Work out the finished part from the listing and answer in its coordinate system (mm). A direction names the side the tool comes from. Give positions to 0.01 mm unless a question says otherwise; leave off trailing zeros.
1) Straight lines are drawn through the part: probe 1 along Y at (x, z) = (0, 6.25) (3 decimals); probe 2 along X at (y, z) = (-9, 5.25); probe 3 along X at (y, z) = (8, 13). For each, find the intervals that lie inside material, in ascending order.
2) Determine the mould class of faces 1 (the face through (-12, 0, 14.1)), 2 (the face through (-19, 3, 12.6)), 3 (the face through (25.865, -10.724, 5.965)) for opening direction X: pulls with the +X half, pulls with the -X half, needs draft (parallel to the pull), parting line crosses it, or undercut.
3) Given pin 1 Ø1 at (y, z) = (-14.5, 11) entering from -X; pin 2 Ø2.5 at (x, y) = (6.5, -18) entering from +Z; pin 3 Ø5 at (y, z) = (-11.5, 11.5) entering from -X, each flat-ended and moving along its own axis, determine where each tip first touches the part or whether it passes through.
4) A tool of negligible diameter and unlimited length cuts with its end or side. For faces 4 (the face through (0, 20, 12.6)), 5 (the face through (-8.2, 7.52, 6.95)), from which of +Z, -Z, +X, -X, +Y, -Y can it reach the whole face along a straight path? Write none if from no direction.
```python
from build123d import *

# Parameters (mm, degrees)
F0_R     = 28
F0_R_2   = 11.125
F1_DEPTH = 14.1
F2_R     = 2
F3_R     = 5
F4_DEPTH = 1.5


# Not quite as in the source:
# - a fillet or chamfer that OpenCascade refuses, or shapes differently, is made with other operations: its cross-section is extruded or revolved along the edge and cut away or added


with BuildPart() as f1:
    # F0 (on Top) → F1 (new body)
    with BuildSketch(Plane.XY):
        Circle(F0_R)
        Circle(F0_R_2, mode=Mode.SUBTRACT)
    extrude(amount=F1_DEPTH)

    # F2
    f2_edges = [f1.edges().sort_by_distance(p)[0] for p in [
        (-28, 0, 14.1),
    ]]
    fillet(f2_edges, radius=F2_R)

    # F3 (on face) → F4 (cut)
    with BuildSketch(Plane.XY.offset(14.1)):
        with Locations((0, 19.5)):
            Circle(F3_R)
        with Locations((-12.5343583889, 14.9378666408)):
            Circle(F3_R)
        with Locations((-19.2037511837, 3.3861394645)):
            Circle(F3_R)
        with Locations((-16.8874953738, -9.75)):
            Circle(F3_R)
        with Locations((-6.6693927949, -18.3240061053)):
            Circle(F3_R)
        with Locations((6.6693927949, -18.3240061053)):
            Circle(F3_R)
        with Locations((16.8874953738, -9.75)):
            Circle(F3_R)
        with Locations((19.2037511837, 3.3861394645)):
            Circle(F3_R)
        with Locations((12.5343583889, 14.9378666408)):
            Circle(F3_R)
    extrude(amount=-F4_DEPTH, mode=Mode.SUBTRACT)

    # F5: fillet of radius 5 on 9 edges, made by hand

    # F5_s1 → F5_t2 (revolve)
    with BuildSketch(Plane.XZ.offset(-19.5)):
        with BuildLine():
            ThreePointArc((5, 14.1), (3.3657774588, 12.9902277714), (1.4292857857, 12.6))
            Line((1.4292857857, 12.6), (5, 12.6))
            Line((5, 12.6), (5, 14.1))
        make_face()
    revolve(axis=Axis((0, 19.5, 12.6), (0, 0, 1)))

    # F5_s3 → F5_t4 (revolve)
    with BuildSketch(Plane.XZ.offset(-14.9378666408)):
        with BuildLine():
            ThreePointArc((-7.5343583889, 14.1), (-9.1685809301, 12.9902277714), (-11.1050726032, 12.6))
            Line((-11.1050726032, 12.6), (-7.5343583889, 12.6))
            Line((-7.5343583889, 12.6), (-7.5343583889, 14.1))
        make_face()
    revolve(axis=Axis((-12.5343583889, 14.9378666408, 12.6), (0, 0, 1)))

    # F5_s5 → F5_t6 (revolve)
    with BuildSketch(Plane.XZ.offset(-3.3861394645)):
        with BuildLine():
            ThreePointArc((-14.2037511837, 14.1), (-15.8379737249, 12.9902277714), (-17.774465398, 12.6))
            Line((-17.774465398, 12.6), (-14.2037511837, 12.6))
            Line((-14.2037511837, 12.6), (-14.2037511837, 14.1))
        make_face()
    revolve(axis=Axis((-19.2037511837, 3.3861394645, 12.6), (0, 0, 1)))

    # F5_s7 → F5_t8 (revolve)
    with BuildSketch(Plane.XZ.offset(9.75)):
        with BuildLine():
            ThreePointArc((-11.8874953738, 14.1), (-13.521717915, 12.9902277714), (-15.4582095881, 12.6))
            Line((-15.4582095881, 12.6), (-11.8874953738, 12.6))
            Line((-11.8874953738, 12.6), (-11.8874953738, 14.1))
        make_face()
    revolve(axis=Axis((-16.8874953738, -9.75, 12.6), (0, 0, 1)))

    # F5_s9 → F5_t10 (revolve)
    with BuildSketch(Plane.XZ.offset(18.3240061053)):
        with BuildLine():
            ThreePointArc((-1.6693927949, 14.1), (-3.303615336, 12.9902277714), (-5.2401070091, 12.6))
            Line((-5.2401070091, 12.6), (-1.6693927949, 12.6))
            Line((-1.6693927949, 12.6), (-1.6693927949, 14.1))
        make_face()
    revolve(axis=Axis((-6.6693927949, -18.3240061053, 12.6), (0, 0, 1)))

    # F5_s11 → F5_t12 (revolve)
    with BuildSketch(Plane.XZ.offset(18.3240061053)):
        with BuildLine():
            ThreePointArc((11.6693927949, 14.1), (10.0351702537, 12.9902277714), (8.0986785806, 12.6))
            Line((8.0986785806, 12.6), (11.6693927949, 12.6))
            Line((11.6693927949, 12.6), (11.6693927949, 14.1))
        make_face()
    revolve(axis=Axis((6.6693927949, -18.3240061053, 12.6), (0, 0, 1)))

    # F5_s13 → F5_t14 (revolve)
    with BuildSketch(Plane.XZ.offset(9.75)):
        with BuildLine():
            ThreePointArc((21.8874953738, 14.1), (20.2532728326, 12.9902277714), (18.3167811595, 12.6))
            Line((18.3167811595, 12.6), (21.8874953738, 12.6))
            Line((21.8874953738, 12.6), (21.8874953738, 14.1))
        make_face()
    revolve(axis=Axis((16.8874953738, -9.75, 12.6), (0, 0, 1)))

    # F5_s15 → F5_t16 (revolve)
    with BuildSketch(Plane.XZ.offset(-3.3861394645)):
        with BuildLine():
            ThreePointArc((24.2037511837, 14.1), (22.5695286426, 12.9902277714), (20.6330369695, 12.6))
            Line((20.6330369695, 12.6), (24.2037511837, 12.6))
            Line((24.2037511837, 12.6), (24.2037511837, 14.1))
        make_face()
    revolve(axis=Axis((19.2037511837, 3.3861394645, 12.6), (0, 0, 1)))

    # F5_s17 → F5_t18 (revolve)
    with BuildSketch(Plane.XZ.offset(-14.9378666408)):
        with BuildLine():
            ThreePointArc((17.5343583889, 14.1), (15.9001358477, 12.9902277714), (13.9636441746, 12.6))
            Line((13.9636441746, 12.6), (17.5343583889, 12.6))
            Line((17.5343583889, 12.6), (17.5343583889, 14.1))
        make_face()
    revolve(axis=Axis((12.5343583889, 14.9378666408, 12.6), (0, 0, 1)))


solid = f1.part
```
Results:
1. probe 1: y = -28 to -11.125, 11.125 to 28
1. probe 2: x = -26.51 to -6.54, 6.54 to 26.51
1. probe 3: x = -26.61 to -7.73, 7.73 to 26.61
2. face 1: needs draft
2. face 2: undercut
2. face 3: parting line crosses it
3. pin 1: stops at x = -24.25
3. pin 2: stops at z = 12.6
3. pin 3: stops at x = -26.51
4. face 4: +Z
4. face 5: +Z, -Z
